```python
from build123d import *

# Parameters (mm, degrees)
SKETCH_1_W      = 90
SKETCH_1_H      = 90
EXTRUDE_1_DEPTH = 6
SKETCH_2_R      = 28
EXTRUDE_2_DEPTH = 95
SKETCH_3_W      = 90
SKETCH_3_H      = 38
EXTRUDE_3_DEPTH = 20


with BuildPart() as part:
    # 草图1 → 凸台-拉伸1 (new body)
    with BuildSketch(Plane.XY):
        Rectangle(SKETCH_1_W, SKETCH_1_H)
    extrude(amount=EXTRUDE_1_DEPTH)

    # 草图2 → 凸台-拉伸2 (add)
    with BuildSketch(Plane.XY):
        Circle(SKETCH_2_R)
    extrude(amount=EXTRUDE_2_DEPTH)

    # 草图3 → 凸台-拉伸3 (add)
    with BuildSketch(Plane.XY):
        with Locations((0, -46)):
            Rectangle(SKETCH_3_W, SKETCH_3_H)
    extrude(amount=EXTRUDE_3_DEPTH)


solid = part.part
```
Design review of the part built by this model. Coordinates are the model's own, in mm. Round coordinates to 2 decimals unless told otherwise and drop trailing zeros. Order: outer loops, then holes, each group sorted by start corner. A loop starts at its lowest first (then second) coordinate and runs counter-clockwise, first axis right, second up. Notation, with made-up numbers: (0.5, 18.5) - (23.5, 18.5) arc R18 cw to (23.5, 53.5) - close; hole circle Ø11 at (-18, 8.25). An arc over 180 degrees is marked (long way). One line per question, with ' | ' between items.
Item 1: Take a section at D-D, the plane x = -36.5. Write out the cut boundary in (y, z).
Checks:
outline: (-65, 0) - (45, 0) - (45, 6) - (-27, 6) - (-27, 20) - (-65, 20) - close
Item 2: Take a section at C-C, the plane z = 43.5. Write out the cut boundary in (x, y), then the cut area to 3 significant figures.
Checks:
outline: circle Ø56 at (0, 0) | area: 2,460 mm²
Item 3: Take a section at A-A, the plane x = 0. Write out the cut boundary in (y, z).
Checks:
outline: (-65, 0) - (45, 0) - (45, 6) - (28, 6) - (28, 95) - (-28, 95) - (-28, 20) - (-65, 20) - close
Item 4: Take a section at B-B, the plane y = 0. Write out the cut boundary in (x, z).
Checks:
outline: (-45, 0) - (45, 0) - (45, 6) - (28, 6) - (28, 95) - (-28, 95) - (-28, 6) - (-45, 6) - close
Item 5: Draft analysis for pull direction Y (two halves, no side actions). For faces 1 (the face through (-26, -27, 13)), 2 (the face through (-1, 45, 3)), 3 (the face through (-45, -23, 5)), 4 (the face through (26, -27, 13)), state which applies: +Y half, -Y half, draft (parallel to the pull), parting line (faces both ways), or undercut.
Checks:
face 1: undercut | face 2: +Y half | face 3: draft | face 4: undercut
Item 6: Wall thickness on line 1 (Z direction, x = 36, y = -58.5); line 2 (Z direction, x = 34, y = 14.5); line 3 (Y direction, x = 41.5, z = 7): over which ranges is each line inside the solid? List them lowest first. Write a range as [from, to].
Checks:
line 1: [0, 20] | line 2: [0, 6] | line 3: [-65, -27]
Item 7: For P1, Ø3, axis at y = -8.5, z = 46, coming from the +X side; P2, Ø1.5, axis at x = 30, z = 70, coming from the +Y side; P3, Ø5, axis at y = -27, z = 70.5, coming from the -X side; P4, Ø11.5, axis at x = 8.5, y = -54, coming from the +Z side, all flat-tipped, find the tip position at first contact; note any pin that passes through.
Checks:
P1: x = 27.11 | P2: through | P3: x = -13.56 | P4: z = 20
